Geometry check sheet. Reference: the model listing, model coordinates, mm. Face numbers are marked on the shaded views. A direction names the side the tool comes from. Give positions to 0.01 mm unless a question says otherwise; leave off trailing zeros. Loops run counter-clockwise (first coordinate to the right, second up) from the corner with the lowest first, then second, coordinate; pieces in that order, holes last. Notation, with made-up numbers: (-24.5, 18.5) -> (-9.5, 18.5) arc R13 cw to (-9.5, 37.5) -> close; hole circle Ø2 at (37.25, 53.5). An arc over 180 degrees is marked (long way). Answer as a JSON object with one key per item and string values.
from build123d import *

# Parameters (mm, degrees)
F1_DEPTH     = 4
F2_T1_DEPTH  = 109.1
F2_T3_DEPTH  = 50
F2_T6_ANGLE  = 90
F2_T8_ANGLE  = 90
F2_T10_ANGLE = 90
F2_T12_ANGLE = 90
F3_R         = 1
F4_W         = 10.7876481488
F4_H         = 3.5392509308
F5_DEPTH     = 3.9
F6_DEPTH     = 4.8
F7_DEPTH     = 5
F8_R         = 1.0596630805
F9_DEPTH     = 18
F10_DEPTH    = 18
F11_R        = 1


# Not quite as in the source:
# - a fillet or chamfer that OpenCascade refuses, or shapes differently, is made with other operations: its cross-section is extruded or revolved along the edge and cut away or added


with BuildPart() as f1:
    # F0 (on Top) → F1 (new body)
    with BuildSketch(Plane.XY):
        with BuildLine():
            Line((26.0500038445, 123.900002712), (-23.9499961555, 123.900002712))
            ThreePointArc((-23.9499961555, 123.900002712), (-29.1472309972, 121.7472375537), (-31.2999961555, 116.550002712))
            Line((-31.2999961555, 116.550002712), (-31.2999961555, 7.450002712))
            ThreePointArc((-31.2999961555, 7.450002712), (-29.1472309972, 2.2527678703), (-23.9499961555, 0.100002712))
            Line((-23.9499961555, 0.100002712), (26.0500038445, 0.100002712))
            ThreePointArc((26.0500038445, 0.100002712), (31.2472386862, 2.2527678703), (33.4000038445, 7.450002712))
            Line((33.4000038445, 7.450002712), (33.4000038445, 116.550002712))
            ThreePointArc((33.4000038445, 116.550002712), (31.2472386862, 121.7472375537), (26.0500038445, 123.900002712))
        make_face()
    extrude(amount=F1_DEPTH)

    # F2: fillet of radius 5 on 1 edges, made by hand

    # F2_s2 → F2_t1 (cut)
    with BuildSketch(Plane.XZ.offset(-116.550002712)):
        with BuildLine():
            ThreePointArc((33.4000038445, 0), (31.6633020191, 2.8729833462), (28.5010243589, 4))
            Line((28.5010243589, 4), (28.5010243589, 4.1))
            Line((28.5010243589, 4.1), (33.4000038445, 4.1))
            Line((33.4000038445, 4.1), (33.5000038445, 4))
            ThreePointArc((33.5000038445, 4), (33.5000038445, 2), (33.4979834342, 0.02))
            Line((33.4979834342, 0.02), (33.4000038445, 0))
        make_face()
        with BuildLine():
            ThreePointArc((-31.2999961555, 0), (-29.5632943301, 2.8729833462), (-26.4010166699, 4))
            Line((-26.4010166699, 4), (-26.4010166699, 4.1))
            Line((-26.4010166699, 4.1), (-31.2999961555, 4.1))
            Line((-31.2999961555, 4.1), (-31.3999961555, 4))
            ThreePointArc((-31.3999961555, 4), (-31.3999961555, 2), (-31.3979757452, 0.02))
            Line((-31.3979757452, 0.02), (-31.2999961555, 0))
        make_face()
    extrude(amount=F2_T1_DEPTH, mode=Mode.SUBTRACT)

    # F2_s4 → F2_t3 (cut)
    with BuildSketch(Plane.YZ.offset(-23.9499961555)):
        with BuildLine():
            ThreePointArc((123.900002712, 0), (122.1633008866, 2.8729833462), (119.0010232264, 4))
            Line((119.0010232264, 4), (119.0010232264, 4.1))
            Line((119.0010232264, 4.1), (123.900002712, 4.1))
            Line((123.900002712, 4.1), (124.000002712, 4))
            ThreePointArc((124.000002712, 4), (124.000002712, 2), (123.9979823017, 0.02))
            Line((123.9979823017, 0.02), (123.900002712, 0))
        make_face()
        with BuildLine():
            ThreePointArc((0.100002712, 0), (1.8367045374, 2.8729833462), (4.9989821976, 4))
            Line((4.9989821976, 4), (4.9989821976, 4.1))
            Line((4.9989821976, 4.1), (0.100002712, 4.1))
            Line((0.100002712, 4.1), (2.712e-06, 4))
            ThreePointArc((2.712e-06, 4), (2.712e-06, 2), (0.0020231223, 0.02))
            Line((0.0020231223, 0.02), (0.100002712, 0))
        make_face()
    extrude(amount=F2_T3_DEPTH, mode=Mode.SUBTRACT)

    # F2_s5 → F2_t6 (revolve, cut)
    with BuildSketch(Plane.YZ.offset(26.0500038445)):
        with BuildLine():
            ThreePointArc((0.100002712, 0), (1.8367045374, 2.8729833462), (4.9989821976, 4))
            Line((4.9989821976, 4), (4.9989821976, 4.1))
            Line((4.9989821976, 4.1), (0.100002712, 4.1))
            Line((0.100002712, 4.1), (2.712e-06, 4))
            ThreePointArc((2.712e-06, 4), (2.712e-06, 2), (0.0020231223, 0.02))
            Line((0.0020231223, 0.02), (0.100002712, 0))
        make_face()
    revolve(axis=Axis((26.0500038445, 7.450002712, 4), (0, 0, 1)), revolution_arc=F2_T6_ANGLE, mode=Mode.SUBTRACT)

    # F2_s7 → F2_t8 (revolve, cut)
    with BuildSketch(Plane.XZ.offset(-116.550002712)):
        with BuildLine():
            ThreePointArc((33.4000038445, 0), (31.6633020191, 2.8729833462), (28.5010243589, 4))
            Line((28.5010243589, 4), (28.5010243589, 4.1))
            Line((28.5010243589, 4.1), (33.4000038445, 4.1))
            Line((33.4000038445, 4.1), (33.5000038445, 4))
            ThreePointArc((33.5000038445, 4), (33.5000038445, 2), (33.4979834342, 0.02))
            Line((33.4979834342, 0.02), (33.4000038445, 0))
        make_face()
    revolve(axis=Axis((26.0500038445, 116.550002712, 4), (0, 0, 1)), revolution_arc=F2_T8_ANGLE, mode=Mode.SUBTRACT)

    # F2_s9 → F2_t10 (revolve, cut)
    with BuildSketch(Plane.YZ.offset(-23.9499961555)):
        with BuildLine():
            ThreePointArc((123.900002712, 0), (122.1633008866, 2.8729833462), (119.0010232264, 4))
            Line((119.0010232264, 4), (119.0010232264, 4.1))
            Line((119.0010232264, 4.1), (123.900002712, 4.1))
            Line((123.900002712, 4.1), (124.000002712, 4))
            ThreePointArc((124.000002712, 4), (124.000002712, 2), (123.9979823017, 0.02))
            Line((123.9979823017, 0.02), (123.900002712, 0))
        make_face()
    revolve(axis=Axis((-23.9499961555, 116.550002712, 4), (0, 0, 1)), revolution_arc=F2_T10_ANGLE, mode=Mode.SUBTRACT)

    # F2_s11 → F2_t12 (revolve, cut)
    with BuildSketch(Plane.XZ.offset(-7.450002712)):
        with BuildLine():
            ThreePointArc((-31.2999961555, 0), (-29.5632943301, 2.8729833462), (-26.4010166699, 4))
            Line((-26.4010166699, 4), (-26.4010166699, 4.1))
            Line((-26.4010166699, 4.1), (-31.2999961555, 4.1))
            Line((-31.2999961555, 4.1), (-31.3999961555, 4))
            ThreePointArc((-31.3999961555, 4), (-31.3999961555, 2), (-31.3979757452, 0.02))
            Line((-31.3979757452, 0.02), (-31.2999961555, 0))
        make_face()
    revolve(axis=Axis((-23.9499961555, 7.450002712, 4), (0, 0, 1)), revolution_arc=F2_T12_ANGLE, mode=Mode.SUBTRACT)

    # F3
    f3_edges = [f1.edges().sort_by_distance(p)[0] for p in [
        (33.400004, 62.000003, 0),
        (31.247239, 121.747238, 0),
        (1.050004, 123.900003, 0),
        (-29.147231, 121.747238, 0),
        (-31.299996, 62.000003, 0),
        (-29.147231, 2.252768, 0),
        (1.050004, 0.100003, 0),
        (31.247239, 2.252768, 0),
    ]]
    fillet(f3_edges, radius=F3_R)

    # F4 (on Top) → F5 (join)
    with BuildSketch(Plane.XY):
        Rectangle(F4_W, F4_H)
    extrude(amount=F5_DEPTH)

    # F6 (add): a face of the model
    f6_faces = [f1.faces().sort_by_distance(p)[0] for p in [
        (0, 1.7696254654, 3.3586156696),
    ]]
    extrude(f6_faces, amount=F6_DEPTH)

    # F7 (add): a face of the model
    f7_faces = [f1.faces().sort_by_distance(p)[0] for p in [
        (0, -1.7696254654, 1.95),
    ]]
    extrude(f7_faces, amount=F7_DEPTH)

    # F8 (on Right) → F9 (join)
    with BuildSketch(Plane.YZ):
        with Locations((-4.8954286613, 1.9693823997)):
            Circle(F8_R)
    extrude(amount=F9_DEPTH)

    # F8 (on Right) → F10 (join)
    with BuildSketch(Plane.YZ):
        with Locations((-4.8954286613, 1.9693823997)):
            Circle(F8_R)
    extrude(amount=-F10_DEPTH)

    # F11
    f11_edges = [f1.edges().sort_by_distance(p)[0] for p in [
        (5.393824, -1.382815, 3.9),
        (-5.393824, -1.382815, 3.9),
        (0, -6.769625, 3.9),
        (0, -6.769625, 0),
        (5.393824, -2.617372, 0),
        (-5.393824, -2.617372, 0),
    ]]
    fillet(f11_edges, radius=F11_R)


solid = f1.part
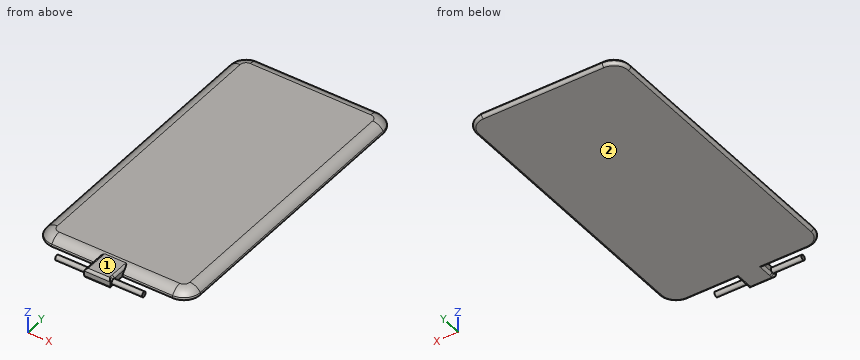
1) Depth check by flat-ended pin: P1, Ø0.6, axis at y = -5, z = 2, coming from the +X side; P2, Ø2, axis at y = 12.5, z = 0.5, coming from the +X side; P3, Ø1.2, axis at y = -6, z = 1.5, coming from the -X side; P4, Ø1.5, axis at y = 0, z = 2.5, coming from the -X side. Enter the tip coordinate at first touch or a pass-through.
Geometry check:
{"P1": "stops at x = 18", "P2": "stops at x = 32.97", "P3": "stops at x = -18", "P4": "stops at x = -5.39"}
2) Material ranges on line 1 along Y through (x, z) = (16, 0.85); line 2 along Y through (x, z) = (-17, 2.6); line 3 along Y through (x, z) = (-16, 1.05), recorded low to high. Write a range as from..to.
Geometry check:
{"line 1": "y = 0.55..123.45", "line 2": "y = -5.75..-4.04, 1.53..122.47", "line 3": "y = -5.42..-4.37, 0.54..123.46"}
3) Section check A-A on y = 62. Record the cut outline in (x, z), plus the area to 3 significant figures.
Geometry check:
{"outline": "(-30.73, 1.5) arc R1 ccw to (-29.87, 0) -> (31.97, 0) arc R1 ccw to (32.83, 1.5) arc R5 ccw to (28.5, 4) -> (-26.4, 4) arc R5 ccw to start", "area": "248 mm2"}
4) Section check B-B on x = -12. Record the cut outline in (y, z).
Geometry check:
{"outline": "circle Ø2.12 at (-4.9, 1.97); (0.67, 1.5) arc R1 ccw to (1.53, 0) -> (122.47, 0) arc R1 ccw to (123.33, 1.5) arc R5 ccw to (119, 4) -> (5, 4) arc R5 ccw to start"}
5) Section check C-C on x = 23.5. Record the cut outline in (y, z).
Geometry check:
{"outline": "(0.67, 1.5) arc R1 ccw to (1.53, 0) -> (122.47, 0) arc R1 ccw to (123.33, 1.5) arc R5 ccw to (119, 4) -> (5, 4) arc R5 ccw to start"}
6) Tool access check on the marked faces 1 and 2. Record the directions out of +Z, -Z, +X, -X, +Y, -Y that give a thin tool (end or side, any length) a straight path to the whole face; none if there is none.
Geometry check:
{"face 1": "+Z, +X, -X, -Y", "face 2": "-Z, +X, -X, +Y, -Y"}
